Geometry check sheet. Reference: drawing and pictorial views, mm from the part's lowest x, y, z. A direction names the side the tool comes from. Coordinates: 2 decimals unless noted, no trailing zeros. Loops run counter-clockwise (first coordinate to the right, second up) from the corner with the lowest first, then second, coordinate; pieces in that order, holes last. Notation, with made-up numbers: (52, 7) -> (93, 7) arc R24 ccw to (93, 28) -> close; hole circle Ø9 at (51, 87.25). An arc over 180 degrees is marked (long way). Answer as a JSON object with one key per item and string values.
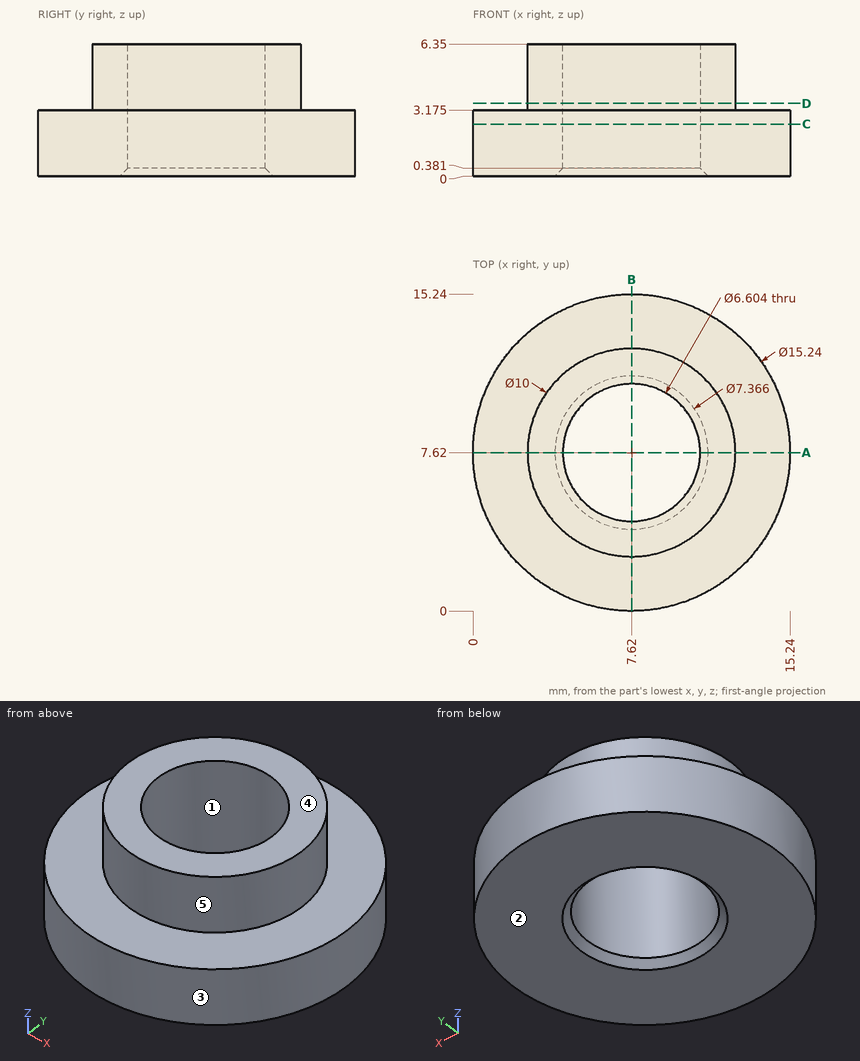
1. Section check D-D, the plane z = 3.5. Record the boundary of the cut face in (x, y).
Evaluation:
{"outline": "circle Ø10 at (7.62, 7.62); hole circle Ø6.6 at (7.62, 7.62)"}
2. Thickness scan on probe 1 along Y at (x, z) = (7.62, 2.85); probe 2 along Y at (x, z) = (10.25, 5); probe 3 along Z at (x, y) = (5.75, 14.25) (3 decimals). Record the ranges inside material, lowest first. Write a range as from..to.
Evaluation:
{"probe 1": "y = 0..4.32, 10.92..15.24", "probe 2": "y = 3.37..5.62, 9.62..11.87", "probe 3": "z = 0..3.175"}
3. Section check C-C, the plane z = 2.5. Record the boundary of the cut face in (x, y).
Evaluation:
{"outline": "circle Ø15.24 at (7.62, 7.62); hole circle Ø6.6 at (7.62, 7.62)"}
4. Tool access check on the marked faces 4 and 5. Record the directions out of +Z, -Z, +X, -X, +Y, -Y that give a thin tool (end or side, any length) a straight path to the whole face; none if there is none.
Evaluation:
{"face 4": "+Z, +X, -X, +Y, -Y", "face 5": "+Z"}
5. Section check A-A, the plane y = 7.62. Record the boundary of the cut face in (x, z) (3 decimals), then the cut area to 3 significant figures.
Evaluation:
{"outline": "(0, 0) -> (3.937, 0) -> (4.318, 0.381) -> (4.318, 6.35) -> (2.62, 6.35) -> (2.62, 3.175) -> (0, 3.175) -> close; (10.922, 0.381) -> (11.303, 0) -> (15.24, 0) -> (15.24, 3.175) -> (12.62, 3.175) -> (12.62, 6.35) -> (10.922, 6.35) -> close", "area": "38.1 mm^2"}
6. Depth check by flat-ended pin: P1, Ø3, axis at x = 2, z = 3.5, coming from the -Y side; P2, Ø2, axis at x = 9, z = 3, coming from the -Y side; P3, Ø4, axis at x = 12.5, y = 2, coming from the +Z side (3 decimals). Enter the tip coordinate at first touch or a pass-through.
Evaluation:
{"P1": "stops at y = 1.23", "P2": "stops at y = 0.01", "P3": "stops at z = 3.175"}
7. Mould release check, pull along Y, two halves, no side actions. Record for the marked faces 1, 2 and 3: released by +Y, released by -Y, zero draft, split by the parting line, or undercut.
Evaluation:
{"face 1": "undercut", "face 2": "zero draft", "face 3": "split by the parting line"}
